from build123d import *

# Parameters (mm, degrees)
F0_R     = 2.5
F0_W     = 21.5
F0_H     = 48.2
F1_DEPTH = 5
F2_SIZE  = 1
F3_SIZE  = 1


with BuildPart() as f1:
    # F0 (on Top) → F1 (new body)
    with BuildSketch(Plane.XY):
        with BuildLine():
            Line((74.005723, 30), (-75.4411, 30))
            ThreePointArc((-75.4411, 30), (-105.4411, 0), (-75.4411, -30))
            Line((-75.4411, -30), (74.005723, -30))
            ThreePointArc((74.005723, -30), (104.005723, 0), (74.005723, 30))
        make_face()
        with Locations((-97.871438, 0)):
            Circle(F0_R, mode=Mode.SUBTRACT)
        with Locations((-39.75, 0)):
            Rectangle(F0_W, F0_H, mode=Mode.SUBTRACT)
        with Locations((-13.25, 0)):
            Rectangle(F0_W, F0_H, mode=Mode.SUBTRACT)
        with Locations((13.25, 0)):
            Rectangle(F0_W, F0_H, mode=Mode.SUBTRACT)
        with Locations((39.75, 0)):
            Rectangle(F0_W, F0_H, mode=Mode.SUBTRACT)
        with Locations((97.871438, 0)):
            Circle(F0_R, mode=Mode.SUBTRACT)
    extrude(amount=F1_DEPTH)

    # F2
    f2_edges = [f1.edges().sort_by_distance(p)[0] for p in [
        (-100.371438, 0, 5),
    ]]
    chamfer(f2_edges, length=F2_SIZE)

    # F3
    f3_edges = [f1.edges().sort_by_distance(p)[0] for p in [
        (95.371438, 0, 5),
    ]]
    chamfer(f3_edges, length=F3_SIZE)


solid = f1.part
Source: CAD feature listing. Evaluate the final solid. Frame: model axes, mm. A direction names the side the tool comes from. Coordinates: 2 decimals unless noted, no trailing zeros. Order: outer loops, then holes, each group sorted by start corner. A loop starts at its lowest first (then second) coordinate and runs counter-clockwise, first axis right, second up.
Item 1: Material intervals for line 1 (Y direction, x = -19, z = 0.9); line 2 (X direction, y = 3.5, z = 2.4); line 3 (X direction, y = -6.5, z = 0.25), sorted ascending.
Output values:
line 1: y = -30 to -24.1, 24.1 to 30
line 2: x = -105.24 to -50.5, -29 to -24, -2.5 to 2.5, 24 to 29, 50.5 to 103.8
line 3: x = -104.73 to -50.5, -29 to -24, -2.5 to 2.5, 24 to 29, 50.5 to 103.29
Item 2: Pull-direction query (Y, two-part tool) for faces 3 (the face through (-2, -30, 2)), 4 (the face through (24, 0, 2)), 5 (the face through (-2, 0, 0)); classes: pulls with the +Y half, pulls with the -Y half, needs draft (parallel to the pull), parting line crosses it, or undercut.
Output values:
face 3: pulls with the -Y half
face 4: undercut
face 5: needs draft
Item 3: Cut plane A-A (x = 6.5). Return loops of the section in (y, z).
Output values:
outline: (-30, 0) - (-24.1, 0) - (-24.1, 5) - (-30, 5) - close; (24.1, 0) - (30, 0) - (30, 5) - (24.1, 5) - close
Item 4: First-contact query: P1, Ø1.5, axis at y = -2, z = 3, coming from the -X side; P2, Ø3, axis at y = 8, z = 3, coming from the -X side; P3, Ø6.5, axis at x = -97.87, y = 0, coming from the +Z side; P4, Ø8, axis at x = 53, y = -9, coming from the -Z side. Flat tips, straight axial feed; report the tip coordinate or a pass-through.
Output values:
P1: stops at x = -105.42
P2: stops at x = -104.73
P3: stops at z = 4.75
P4: stops at z = 0
Item 5: Cut plane D-D (y = -10). Return loops of the section in (x, z), plus the area to 3 significant figures.
Output values:
outline: (-103.73, 0) - (-50.5, 0) - (-50.5, 5) - (-103.73, 5) - close; (-29, 0) - (-24, 0) - (-24, 5) - (-29, 5) - close; (-2.5, 0) - (2.5, 0) - (2.5, 5) - (-2.5, 5) - close; (24, 0) - (29, 0) - (29, 5) - (24, 5) - close; (50.5, 0) - (102.29, 0) - (102.29, 5) - (50.5, 5) - close
area: 600 mm2
Item 6: Cut plane B-B (y = 0). Count the separate pieces of the cut face and the enclosed holes in it, plus the area to 3 significant figures.
Output values:
separate pieces: 7
enclosed holes: 0
area: 565 mm2
Item 7: Cut plane C-C (z = 1.45). Return loops of the section in (x, y), plus the area to 3 significant figures.
Output values:
outline: (-75.44, -30) - (74.01, -30) arc R30 ccw to (74.01, 30) - (-75.44, 30) arc R30 ccw to start; hole circle Ø5 at (-97.87, 0); hole (-50.5, -24.1) - (-29, -24.1) - (-29, 24.1) - (-50.5, 24.1) - close; hole (-24, -24.1) - (-2.5, -24.1) - (-2.5, 24.1) - (-24, 24.1) - close; hole (2.5, -24.1) - (24, -24.1) - (24, 24.1) - (2.5, 24.1) - close; hole (29, -24.1) - (50.5, -24.1) - (50.5, 24.1) - (29, 24.1) - close; hole circle Ø5 at (97.87, 0)
area: 7,610 mm2
Item 8: Set-up query: faces 1 (the face through (40, -24.1, 2)), 2 (the face through (-105.434, 0.66, 2.465)). Return all of +Z, -Z, +X, -X, +Y, -Y with unobstructed straight access to the full face (end or side cutting, diameter ignored); none if empty.
Output values:
face 1: +Z, -Z
face 2: +Z, -Z, -X
